Autodesk Inventor part; units mm, degrees
ref_plane "YZ Plane" through (0, 0, 0) normal (1, 0, 0) x (0, 1, 0)
ref_plane "XZ Plane" through (0, 0, 0) normal (0, 1, 0) x (-1, 0, 0)
ref_plane "XY Plane" through (0, 0, 0) normal (0, 0, 1) x (1, 0, 0)
sketch "Sketch1" plane through (0, 0, 0) normal (0, 0, 1) x (1, 0, 0)
  line L0 (-40, 16) -> (40, 16)
  line L1 (40, 16) -> (40, -16)
  line L2 (40, -16) -> (-40, -16)
  line L3 (-40, -16) -> (-40, 16)
  line L4 (-40, 16) -> (40, -16) construction
  line L5 (40, 16) -> (-40, -16) construction
  point P0 (0, 0)
  dimension "d0" = 80
  dimension "d1" = 32
extrude "Extrusion1" add sketch "Sketch1" along normal blind 10
sketch "Sketch2" plane through (0, 0, 10) normal (0, 0, 1) x (1, 0, 0)
  line L0 (-28, 0) -> (-40, 0)
  line L1 (-40, 16) -> (-40, -16)
  line L2 (28, 0) -> (40, 0)
  line L3 (40, -16) -> (40, 16)
  point P0 (0, 0)
  dimension "d4" = 56
hole "Hole1" at (28, 0, 10) at (-28, 0, 10) direction (0, 0, -1) diameter 8.2 end through all
sketch "Sketch4" plane through (0, 0, 0) normal (0, 0, -1) x (-1, 0, 0)
  line L0 (-8.5, 0) -> (-40, 0) construction
  line L1 (8.5, 0) -> (40, 0) construction
  line L2 (40, 16) -> (40, -16)
  line L3 (-40, -16) -> (-40, 16)
  line L4 (-40, 0) -> (40, 0)
  point P0 (0, 0)
  dimension "d13" = 8.5
hole "Hole2" at (-8.5, 0, 0) at (8.5, 0, 0) direction (0, 0, 1) diameter 2.6 end through all counterbore diameter 6.2 counterbore depth 2.2
sketch "Sketch5" plane through (0, 0, 0) normal (0, 0, -1) x (-1, 0, 0)
  point P0 (0, 0)
  point P1 (0, 0)
hole "Hole3" at (0, 0, 0) direction (0, 0, 1) diameter 7.1 end through all counterbore diameter 8 counterbore depth 8.1
properties part number "13042026-09"
Check sheet for the modelled part. Datum: model origin and axes. Units: mm. A direction names the side the tool comes from. Round coordinates to 2 decimals unless told otherwise and drop trailing zeros. Order: outer loops, then holes, each group sorted by start corner. A loop starts at its lowest first (then second) coordinate and runs counter-clockwise, first axis right, second up. Notation, with made-up numbers: (82, -22) - (90, -22) arc R23 ccw to (90, 5) - close; hole circle Ø6 at (-12.5, -24.75). An arc over 180 degrees is marked (long way). Write item = value, one per line.
Q1. Tool access check on faces 1 (the face through (-1, 4, 10)), 2 (the face through (-7, 0, 2.2)). Record the directions out of +Z, -Z, +X, -X, +Y, -Y that give a thin tool (end or side, any length) a straight path to the whole face; none if there is none.
Computed:
face_1 = +Z, +X, -X, +Y, -Y
face_2 = -Z
Q2. Section check A-A (x = 0). Record the boundary of the cut face in (y, z).
Computed:
outline = (-16, 0) - (-4, 0) - (-4, 8.1) - (-3.55, 8.1) - (-3.55, 10) - (-16, 10) - close; (3.55, 8.1) - (4, 8.1) - (4, 0) - (16, 0) - (16, 10) - (3.55, 10) - close
Q3. Draft check along X on faces 3 (the face through (1, -16, 5)), 4 (the face through (5.426, -0.404, 1.115)), 5 (the face through (-40, 0, 5)). Enter one of: pulls with the +X half, pulls with the -X half, needs draft (parallel to the pull), parting line crosses it, or undercut.
Computed:
face_3 = needs draft
face_4 = undercut
face_5 = pulls with the -X half
Q4. Section check B-B (z = 4.5). Record the boundary of the cut face in (x, y).
Computed:
outline = (-40, -16) - (40, -16) - (40, 16) - (-40, 16) - close; hole circle Ø8.2 at (-28, 0); hole circle Ø2.6 at (-8.5, 0); hole circle Ø8 at (0, 0); hole circle Ø2.6 at (8.5, 0); hole circle Ø8.2 at (28, 0)
Q5. Go/stop test with flat-tipped pins: pin 1 (5 mm diameter, centred on x = -28, y = 0, fed in from +Z); pin 2 (5 mm diameter, centred on x = -8.5, y = 0, fed in from -Z). Record where each tip stops, or that it passes through.
Computed:
pin_1 = through
pin_2 = 2.2
Q6. Section check C-C (y = 0). State how many separate pieces and enclosed holes the cut face has, and give its area (3 significant figures).
Computed:
separate_pieces = 6
enclosed_holes = 0
area = 490 mm^2
Q7. Section check D-D (x = 28). Record the boundary of the cut face in (y, z), and give its area (3 significant figures).
Computed:
outline = (-16, 0) - (-4.1, 0) - (-4.1, 10) - (-16, 10) - close; (4.1, 0) - (16, 0) - (16, 10) - (4.1, 10) - close
area = 238 mm^2
Q8. Thickness scan on line 1 along X through (y, z) = (0, 7); line 2 along X through (y, z) = (-2, 7); line 3 along Y through (x, z) = (8.5, 6.5). Record the ranges inside material, lowest first.
Computed:
line_1 = -40 to -32.1, -23.9 to -9.8, -7.2 to -4, 4 to 7.2, 9.8 to 23.9, 32.1 to 40
line_2 = -40 to -31.58, -24.42 to -3.46, 3.46 to 24.42, 31.58 to 40
line_3 = -16 to -1.3, 1.3 to 16
